Job drawing, mm, ordinate dimensions from the low corner. One solid piece. A direction names the side the tool comes from. Round coordinates to 2 decimals unless told otherwise and drop trailing zeros. Loops run counter-clockwise (first coordinate to the right, second up) from the corner with the lowest first, then second, coordinate; pieces in that order, holes last. Notation, with made-up numbers: M 9,83.5 L 47,83.5 A30 ccw 47,117.5 Z; hole C 24,50 d3. An arc over 180 degrees is marked long. Use one line per item in the form item = value. Start each with the question number.
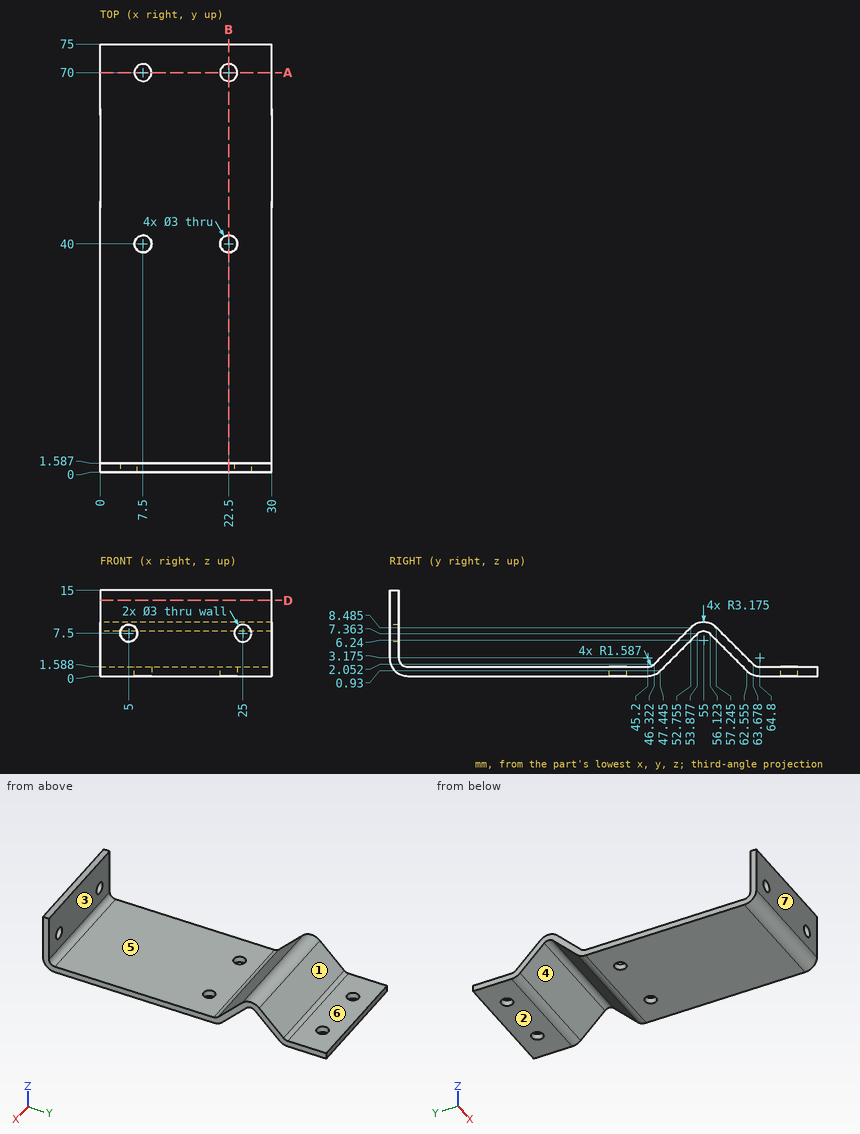
Q1. Saw through at A-A (y = 70). Give the cut face in (x, z).
Q2. Pull direction Y, two halves, no side cores. Call the marked faces 1, 2 and 3: pulls with the +Y half, pulls with the -Y half, needs draft (parallel to the pull), parting line crosses it, or undercut.
Q3. Drop flat-ended pins along their axis: P1, Ø4, axis at x = 22.5, y = 40, coming from the +Z side; P2, Ø10, axis at x = 6, y = 56.5, coming from the -Z side (1 decimal); P3, Ø4, axis at x = 10, y = 62.5, coming from the +Z side. Give the stop position or say it passes through.
Q4. Tool access for the marked faces 4, 5, 6 and 7: list every direction of +Z, -Z, +X, -X, +Y, -Y with a clear straight run to the whole face (end or side of a thin tool).
Q5. Saw through at B-B (x = 22.5). Give the number of separate pieces and of enclosed holes in the cut face, and give its area (3 significant figures).
Q6. Saw through at D-D (z = 13.25). Give the cut face in (x, y).
Q7. Wall check: probe 1 along X at (y, z) = (40, 1.2); probe 2 along Y at (x, z) = (20.5, 2.25) (1 decimal); probe 3 along Y at (x, z) = (5, 3.5) (1 decimal). Give the ranges that are in metal, low to high.
Filled in:
q1.outline = M 0,0 L 6,0 L 6,1.59 L 0,1.59 Z; M 9,0 L 21,0 L 21,1.59 L 9,1.59 Z; M 24,0 L 30,0 L 30,1.59 L 24,1.59 Z
q2.face_1 = pulls with the +Y half
q2.face_2 = needs draft
q2.face_3 = undercut
q3.P1 = 1.59
q3.P2 = 2
q3.P3 = 5.23
q4.face_4 = -Z, +X, -X
q4.face_5 = +Z, +X, -X
q4.face_6 = +Z, +X, -X, +Y
q4.face_7 = +Z, -Z, +X, -X, -Y
q5.separate_pieces = 3
q5.enclosed_holes = 0
q5.area = 139 mm²
q6.outline = M 0,0 L 30,0 L 30,1.59 L 0,1.59 Z
q7.probe_1 = 0 to 6, 9 to 21, 24 to 30
q7.probe_2 = 0.1 to 1.9, 46.5 to 48.8, 61.2 to 63.5
q7.probe_3 = 0 to 1.6, 47.8 to 50, 60 to 62.2
